```python
from build123d import *

# Parameters (mm, degrees)
BOSS_EXTRUDE1_DEPTH = 11
SHELL1_T            = -2
SKETCH3_R           = 0.625
CUT_EXTRUDE1_DEPTH  = 10


with BuildPart() as part:
    # Sketch1 → Boss-Extrude1 (new body)
    with BuildSketch(Plane(origin=(0, 0, 0), x_dir=(1, 0, 0), z_dir=(0, 1, 0))):
        Polygon((0, 0), (5.656854249, -5.656854249), (14.142135624, 2.828427125), (0, 16.970562748), (-14.142135624, 2.828427125), (-5.656854249, -5.656854249), align=None)
    extrude(amount=BOSS_EXTRUDE1_DEPTH)

    # Shell1
    shell1_openings = [part.faces().sort_by_distance(p)[0] for p in [
        (0, 11, -1.885618083),
    ]]
    offset(amount=SHELL1_T, openings=shell1_openings, kind=Kind.INTERSECTION)

    # Sketch3 → Cut-Extrude1 (cut)
    with BuildSketch(Plane.XZ):
        with Locations((-5.656854249, -1.558427125)):
            Circle(SKETCH3_R)
        with Locations((-5.656854249, -4.098427125)):
            Circle(SKETCH3_R)
        with Locations((0, -6.308427125)):
            Circle(SKETCH3_R)
        with Locations((0, -8.848427125)):
            Circle(SKETCH3_R)
        with Locations((5.656854249, -1.558427125)):
            Circle(SKETCH3_R)
        with Locations((5.656854249, -4.098427125)):
            Circle(SKETCH3_R)
    extrude(amount=-CUT_EXTRUDE1_DEPTH, mode=Mode.SUBTRACT)


solid = part.part
```
Geometry: final body of the model. Coordinates: model frame, mm. A direction names the side the tool comes from. Coordinates: 2 decimals unless noted, no trailing zeros. Order: outer loops, then holes, each group sorted by start corner. A loop starts at its lowest first (then second) coordinate and runs counter-clockwise, first axis right, second up. Notation, with made-up numbers: (13, 79) -> (45, 79) arc R23 cw to (45, 96) -> close; hole circle Ø10 at (10, 62.25). An arc over 180 degrees is marked (long way). Write item = value, one per line.
(1) Pin query (flat end, axial travel): pin 1 Ø1 at (y, z) = (9.5, -0.5) entering from -X; pin 2 Ø1.5 at (y, z) = (7.5, 2.5) entering from -X; pin 3 Ø13.5 at (x, z) = (0, -8) entering from +Y; pin 4 Ø6 at (x, y) = (6.5, 4) entering from -Z. Return the tip coordinate at first contact, or that it passes through.
Solved:
pin_1 = -12.31
pin_2 = -9.56
pin_3 = 11
pin_4 = -13.47
(2) Pull-direction query (X, two-part tool) for faces 4 (the flat face through (7.17, 5.42, -9.8)), 5 (the flat face through (-9.959, 5.423, 1.355)), 6 (the cylindrical face through (5.95, 0.99, -4.65)); classes: pulls with the +X half, pulls with the -X half, needs draft (parallel to the pull), parting line crosses it, or undercut.
Solved:
face_4 = pulls with the +X half
face_5 = pulls with the -X half
face_6 = undercut
(3) Cut plane C-C on x = 10.5. Return loops of the section in (y, z).
Solved:
outline = (0, -6.47) -> (11, -6.47) -> (11, -3.64) -> (2, -3.64) -> (2, -2.01) -> (11, -2.01) -> (11, 0.81) -> (0, 0.81) -> close
(4) Cut plane B-B on z = 2.25. Return loops of the section in (x, y), plus the area to 3 significant figures.
Solved:
outline = (-9.06, 0) -> (-2.25, 0) -> (-2.25, 11) -> (-5.08, 11) -> (-5.08, 2) -> (-6.24, 2) -> (-6.24, 11) -> (-9.06, 11) -> close; (2.25, 0) -> (9.06, 0) -> (9.06, 11) -> (6.24, 11) -> (6.24, 2) -> (5.08, 2) -> (5.08, 11) -> (2.25, 11) -> close
area = 129 mm²
(5) Line query: line 1 (Z direction, x = 5.75, y = 1); line 2 (X direction, y = 9.5, z = 1.25); line 3 (Y direction, x = 0, z = -13.5). Output: solid intervals per line, ascending.
Solved:
line_1 = -11.22 to -4.72, -3.48 to -2.18, -0.94 to 5.56
line_2 = -10.06 to -7.24, -4.08 to -1.25, 1.25 to 4.08, 7.24 to 10.06
line_3 = 0 to 2
(6) Cut plane A-A on y = 5.25. Return loops of the section in (x, z).
Solved:
outline = (-14.14, -2.83) -> (0, -16.97) -> (14.14, -2.83) -> (5.66, 5.66) -> (0, 0) -> (-5.66, 5.66) -> close; hole (-11.31, -2.83) -> (0, -14.14) -> (11.31, -2.83) -> (5.66, 2.83) -> (0, -2.83) -> (-5.66, 2.83) -> close
(7) Cut plane D-D on x = -4. Return loops of the section in (y, z), plus the area to 3 significant figures.
Solved:
outline = (0, -12.97) -> (11, -12.97) -> (11, -10.14) -> (2, -10.14) -> (2, 1.17) -> (11, 1.17) -> (11, 4) -> (0, 4) -> close
area = 84.9 mm²
(8) Access query for faces 1 (the flat face through (-3, 5, 3)), 2 (the flat face through (-5.58, 6.44, -8.56)), 3 (the cylindrical face through (0.3, 1, -8.3)). Directions: +Z, -Z, +X, -X, +Y, -Y. A direction counts if a zero-diameter tool reaches every point of the face in a straight line with its end or side. Return the directions, or none.
Solved:
face_1 = +Z, +Y, -Y
face_2 = +Y
face_3 = +Y, -Y
